Build history of the part. All positions in model axes, mm. Face numbers are marked on the shaded views. Give positions to 0.01 mm unless a question says otherwise; leave off trailing zeros. Loops run counter-clockwise (first coordinate to the right, second up) from the corner with the lowest first, then second, coordinate; pieces in that order, holes last.
1) Wall check: line 1 (Y direction, x = 12.7, z = 4) (3 decimals); line 2 (X direction, y = 15, z = 4.75); line 3 (Y direction, x = 11.5, z = 3.25). Give the ranges that are in metal, low to high.
2) Band-saw the part on D-D on x = 21.5. List the corners of the cut face in (y, z).
3) Band-saw the part on B-B on y = 0. List the corners of the cut face in (x, z) (3 decimals), then the cut area to 3 significant figures.
4) Band-saw the part on C-C on z = 1.25. List the corners of the cut face in (x, y) (3 decimals), then the cut area to 3 significant figures.
5) Band-saw the part on A-A on x = -12.7. List the corners of the cut face in (y, z) (3 decimals), then the cut area to 3 significant figures.
6) Flat gauge pin, fed straight in: P1, Ø4, axis at x = 12.7, y = -17.78, coming from the -Z side. Where does the tip first touch, or does it go through?
7) Two-plate mould, pull along Y, no slides. Class the marked faces 1, 2, 3 and 4: +Y half, -Y half, draft (parallel to the pull), parting line (faces both ways), or undercut.
```python
from build123d import *

# Parameters (mm, degrees)
SKETCH2_W           = 50.8
SKETCH2_H           = 68.58
BOSS_EXTRUDE1_DEPTH = 6.35
FILLET1_R           = 7.62
SKETCH5_R           = 3.175
CUT_EXTRUDE1_DEPTH  = 44.142630889
LPATTERN1_COUNT     = 2
LPATTERN1_PITCH     = 17.78
LPATTERN1_COL_COUNT = 2
LPATTERN1_COL_PITCH = 17.78


with BuildPart() as part:
    # Sketch2 → Boss-Extrude1 (new body)
    with BuildSketch(Plane.XY):
        Rectangle(SKETCH2_W, SKETCH2_H)
    extrude(amount=BOSS_EXTRUDE1_DEPTH)

    # Fillet1
    fillet1_edges = [part.edges().sort_by_distance(p)[0] for p in [
        (25.4, -34.29, 3.175),
        (-25.4, -34.29, 3.175),
        (-25.4, 34.29, 3.175),
        (25.4, 34.29, 3.175),
    ]]
    fillet(fillet1_edges, radius=FILLET1_R)

    # Sketch5 → Cut-Extrude1 (cut, through all)
    with BuildSketch(Plane.XY.offset(6.35)):
        with Locations((-12.7, 0)):
            Circle(SKETCH5_R)
        with Locations((12.7, 0)):
            Circle(SKETCH5_R)
    cut_extrude1 = extrude(amount=-CUT_EXTRUDE1_DEPTH, mode=Mode.SUBTRACT)

    # LPattern1: Cut-Extrude1 ×2
    with Locations(*[(0, -i * LPATTERN1_PITCH, 0) for i in range(1, LPATTERN1_COUNT)]):
        add(cut_extrude1, mode=Mode.SUBTRACT)

    # LPattern1 col: Cut-Extrude1 ×2
    with Locations(*[(0, i * LPATTERN1_COL_PITCH, 0) for i in range(1, LPATTERN1_COL_COUNT)]):
        add(cut_extrude1, mode=Mode.SUBTRACT)


solid = part.part
```
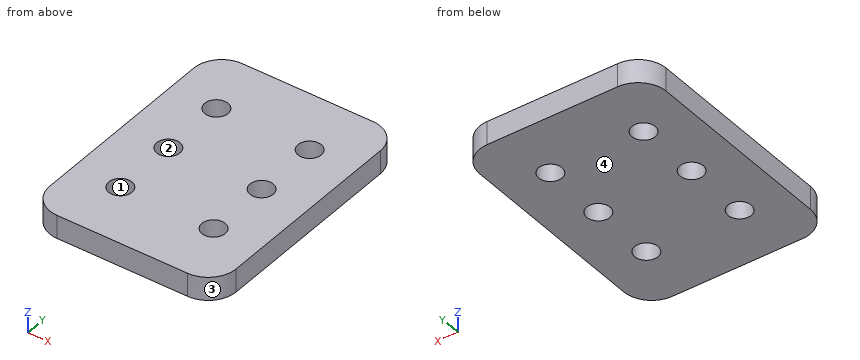
Findings below:
1. line 1: y = -34.29 to -20.955, -14.605 to -3.175, 3.175 to 14.605, 20.955 to 34.29
1. line 2: x = -25.4 to -14.23, -11.17 to 11.17, 14.23 to 25.4
1. line 3: y = -34.29 to -20.72, -14.84 to -2.94, 2.94 to 14.84, 20.72 to 34.29
2. outline: (-33.32, 0) - (33.32, 0) - (33.32, 6.35) - (-33.32, 6.35) - close
3. outline: (-25.4, 0) - (-15.875, 0) - (-15.875, 6.35) - (-25.4, 6.35) - close; (-9.525, 0) - (9.525, 0) - (9.525, 6.35) - (-9.525, 6.35) - close; (15.875, 0) - (25.4, 0) - (25.4, 6.35) - (15.875, 6.35) - close
3. area: 242 mm2
4. outline: (-25.4, -26.67) arc R7.62 ccw to (-17.78, -34.29) - (17.78, -34.29) arc R7.62 ccw to (25.4, -26.67) - (25.4, 26.67) arc R7.62 ccw to (17.78, 34.29) - (-17.78, 34.29) arc R7.62 ccw to (-25.4, 26.67) - close; hole circle Ø6.35 at (-12.7, -17.78); hole circle Ø6.35 at (-12.7, 0); hole circle Ø6.35 at (-12.7, 17.78); hole circle Ø6.35 at (12.7, -17.78); hole circle Ø6.35 at (12.7, 0); hole circle Ø6.35 at (12.7, 17.78)
4. area: 3,240 mm2
5. outline: (-34.29, 0) - (-20.955, 0) - (-20.955, 6.35) - (-34.29, 6.35) - close; (-14.605, 0) - (-3.175, 0) - (-3.175, 6.35) - (-14.605, 6.35) - close; (3.175, 0) - (14.605, 0) - (14.605, 6.35) - (3.175, 6.35) - close; (20.955, 0) - (34.29, 0) - (34.29, 6.35) - (20.955, 6.35) - close
5. area: 315 mm2
6. P1: passes through
7. face 1: undercut
7. face 2: undercut
7. face 3: -Y half
7. face 4: draft
